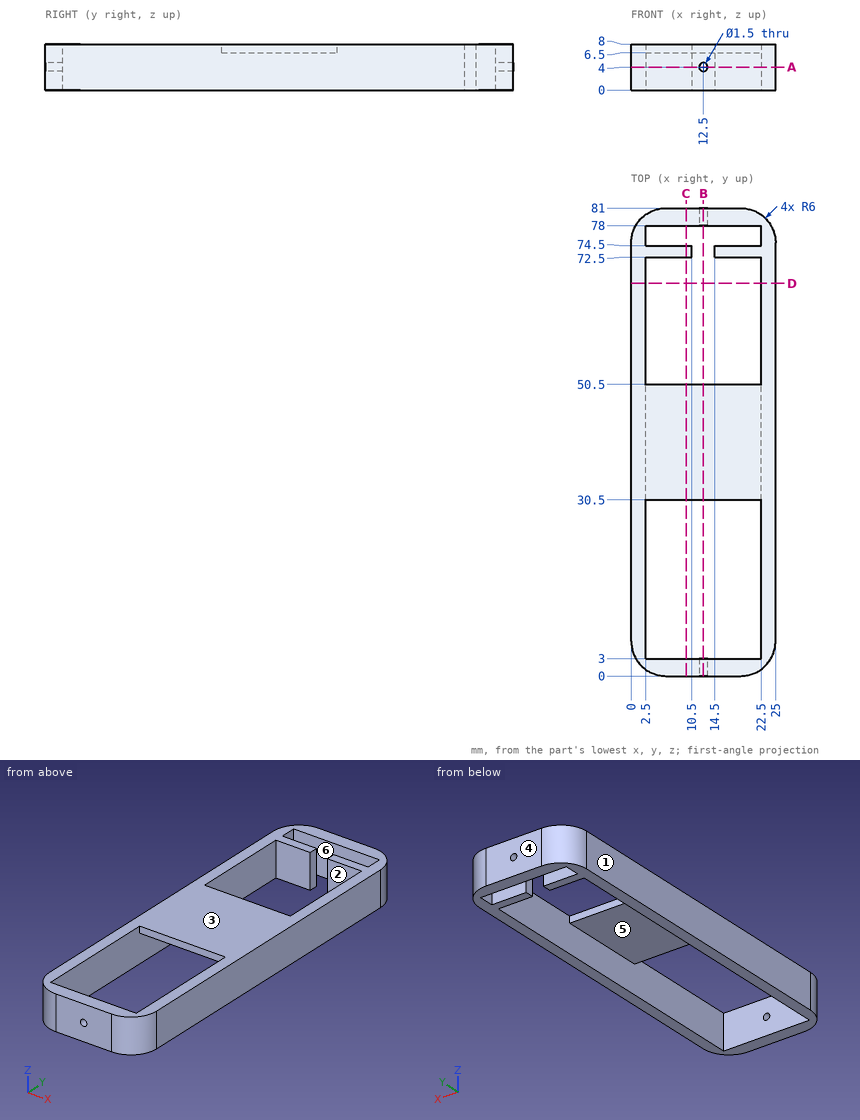
The drawing under review shows one solid part. Ordinate dimensions are in mm from its lowest x, y, z. A direction names the side the tool comes from. Coordinates: 2 decimals unless noted, no trailing zeros. Order: outer loops, then holes, each group sorted by start corner. A loop starts at its lowest first (then second) coordinate and runs counter-clockwise, first axis right, second up. Notation, with made-up numbers: M 70.5,65 L 80.5,65 A20 cw 80.5,71 Z; hole C 70.5,84.5 d1. An arc over 180 degrees is marked long. Use a Markdown table: item, result.
(1) For P1, Ø10, axis at x = 9.5, y = 45.5, coming from the -Z side, flat-tipped, find the tip position at first contact; note if it passes through.
Worked answers:
| item | result |
|---|---|
| P1 | stops at z = 6.5 |
(2) Add section A-A (z = 4). Give the boundary of the cut face in (x, y).
Worked answers:
| item | result |
|---|---|
| outline | M 0,6 A6 ccw 6,0 L 11.75,0 L 11.75,3 L 2.5,3 L 2.5,72.5 L 10.5,72.5 L 10.5,74.5 L 2.5,74.5 L 2.5,78 L 11.75,78 L 11.75,81 L 6,81 A6 ccw 0,75 Z; M 13.25,0 L 19,0 A6 ccw 25,6 L 25,75 A6 ccw 19,81 L 13.25,81 L 13.25,78 L 22.5,78 L 22.5,74.5 L 14.5,74.5 L 14.5,72.5 L 22.5,72.5 L 22.5,3 L 13.25,3 Z |
(3) For the marked faces 4, 5 and 6, list the 3-axis set-ups (+Z, -Z, +X, -X, +Y, -Y) from which the entire face can be reached by the end or side of a thin tool; tool diameter is ignored.
Worked answers:
| item | result |
|---|---|
| face 4 | +Z, -Z, +X, -X, +Y |
| face 5 | -Z |
| face 6 | +Z, -Z |
(4) Wall thickness on probe 1 along Y at (x, z) = (17.25, 7); probe 2 along Z at (x, y) = (12.5, 78.65); probe 3 along Y at (x, z) = (6, 5.75): over which ranges is each line inside the solid? List them lowest first.
Worked answers:
| item | result |
|---|---|
| probe 1 | y = 0 to 3, 30.5 to 50.5, 72.5 to 74.5, 78 to 81 |
| probe 2 | z = 0 to 3.25, 4.75 to 8 |
| probe 3 | y = 0 to 3, 72.5 to 74.5, 78 to 81 |
(5) Add section C-C (x = 9.5). Give the boundary of the cut face in (y, z).
Worked answers:
| item | result |
|---|---|
| outline | M 0,0 L 3,0 L 3,8 L 0,8 Z; M 30.5,6.5 L 50.5,6.5 L 50.5,8 L 30.5,8 Z; M 72.5,0 L 74.5,0 L 74.5,8 L 72.5,8 Z; M 78,0 L 81,0 L 81,8 L 78,8 Z |
(6) Add section D-D (y = 68). Give the boundary of the cut face in (x, z), then the cut area to 3 significant figures.
Worked answers:
| item | result |
|---|---|
| outline | M 0,0 L 2.5,0 L 2.5,8 L 0,8 Z; M 22.5,0 L 25,0 L 25,8 L 22.5,8 Z |
| area | 40.0 mm2 |
(7) Draft analysis for pull direction X (two halves, no side actions). For the marked faces 1, 2 and 3, state which applies: released by +X, released by -X, zero draft, split by the parting line, or undercut.
Worked answers:
| item | result |
|---|---|
| face 1 | released by -X |
| face 2 | undercut |
| face 3 | zero draft |
(8) Add section B-B (x = 12.5). Give the boundary of the cut face in (y, z).
Worked answers:
| item | result |
|---|---|
| outline | M 0,0 L 3,0 L 3,3.25 L 0,3.25 Z; M 0,4.75 L 3,4.75 L 3,8 L 0,8 Z; M 30.5,6.5 L 50.5,6.5 L 50.5,8 L 30.5,8 Z; M 78,0 L 81,0 L 81,3.25 L 78,3.25 Z; M 78,4.75 L 81,4.75 L 81,8 L 78,8 Z |
